```python
from build123d import *

# Parameters (mm, degrees)
SKETCH_1_W           = 88
SKETCH_1_H           = 35
EXTRUDE_1_DEPTH      = 4
EXTRUDE_1_DEPTH_BACK = 4
SKETCH_2_R           = 1.5
CUT_EXTRUDE_1_DEPTH  = 36
EXTRUDE_2_DEPTH      = 12.5


with BuildPart() as part:
    # Sketch 1 → Extrude 1 (new body, two sides)
    with BuildSketch(Plane(origin=(0, 0, 0), x_dir=(1, 0, 0), z_dir=(0, 1, 0))) as extrude_1_sk:
        Rectangle(SKETCH_1_W, SKETCH_1_H)
    extrude(amount=EXTRUDE_1_DEPTH)
    extrude(extrude_1_sk.sketch, amount=-EXTRUDE_1_DEPTH_BACK)

    # Sketch 2 → Cut-Extrude 1 (cut, through all)
    with BuildSketch(Plane(origin=(0, 0, -17.5), x_dir=(-1, 0, 0), z_dir=(0, 0, -1))):
        with Locations((39, 0)):
            Circle(SKETCH_2_R)
        with Locations((-39, 0)):
            Circle(SKETCH_2_R)
        with Locations((-9, 0)):
            Circle(SKETCH_2_R)
        with Locations((9, 0)):
            Circle(SKETCH_2_R)
    extrude(amount=-CUT_EXTRUDE_1_DEPTH, mode=Mode.SUBTRACT)

    # Sketch 3 → Extrude 2 (add, symmetric)
    with BuildSketch(Plane.XY):
        Polygon((29, 4), (22.07179677, 16), (-13.215390309, 16), (-34, 4), align=None)
    extrude(amount=EXTRUDE_2_DEPTH, both=True)


solid = part.part
```
Design review of the part built by this model. Coordinates are the model's own, in mm. A direction names the side the tool comes from. Give positions to 0.01 mm unless a question says otherwise; leave off trailing zeros. Order: outer loops, then holes, each group sorted by start corner. A loop starts at its lowest first (then second) coordinate and runs counter-clockwise, first axis right, second up. Notation, with made-up numbers: M 31.25,44.5 L 62.25,44.5 A27 cw 62.25,68.5 Z; hole C 62,38 d6. An arc over 180 degrees is marked long. One line per question, with ' | ' between items. Start each with the question number.
Q1. For pin 1 Ø9.5 at (x, y) = (7, 8.5) entering from -Z; pin 2 Ø2 at (y, z) = (5.5, 4) entering from +X; pin 3 Ø2 at (y, z) = (9, -11) entering from -X; pin 4 Ø5 at (y, z) = (7, -6.5) entering from -X, all flat-tipped, find the tip position at first contact; note any pin that passes through.
Q2. We need section D-D (x = 9). Write out the cut boundary in (y, z).
Q3. For L1, parallel to Y at x = -9, z = 1; L2, parallel to X at y = -1.25, z = 16.5; L3, parallel to Z at x = -10, y = 5.75, list the stretches that pass through material, from the lowest coordinate up. Write a range as [from, to].
Q4. We need section B-B (z = 4.5). Write out the cut boundary in (x, y).
Q5. The part is to be moulded in two halves that separate along Y. For faces 6 (the face through (-37.8, -0.9, -0.2)), 7 (the face through (10.5, 0.07, -0.25)), 8 (the face through (-1, 0, -17.5)), 9 (the face through (-1, -4, 0)), say which applies: +Y half, -Y half, draft (parallel to the pull), parting line (faces both ways), or undercut.
Q6. We need section A-A (x = -39). Write out the cut boundary in (y, z), plus the area to 3 significant figures.
Q7. We need section C-C (x = -3.5). Write out the cut boundary in (y, z).
Q8. Machinability: for faces 1 (the face through (4, 9, 12.5)), 2 (the face through (25.58, 9.92, 0.18)), 3 (the face through (-1, 4, 15)), 4 (the face through (-1, 0, 17.5)), 5 (the face through (4, 9, -12.5)), which of the approach directions +Z, -Z, +X, -X, +Y, -Y give a long, thin tool a straight path to every point of the face, cutting with its end or side? Answer none if there is none.
Returned:
1) pin 1: z = -17.5 | pin 2: x = 28.71 | pin 3: x = -27.07 | pin 4: x = -33.13
2) outline: M -4,-17.5 L -1.5,-17.5 L -1.5,17.5 L -4,17.5 Z; M 1.5,-17.5 L 4,-17.5 L 4,-12.5 L 16,-12.5 L 16,12.5 L 4,12.5 L 4,17.5 L 1.5,17.5 Z
3) L1: [-4, -1.5], [1.5, 16] | L2: [-44, -39.83], [-38.17, -9.83], [-8.17, 8.17], [9.83, 38.17], [39.83, 44] | L3: [-12.5, 12.5]
4) outline: M -44,-4 L 44,-4 L 44,4 L 29,4 L 22.07,16 L -13.22,16 L -34,4 L -44,4 Z; hole C -39,0 d3; hole C -9,0 d3; hole C 9,0 d3; hole C 39,0 d3
5) face 6: undercut | face 7: undercut | face 8: draft | face 9: -Y half
6) outline: M -4,-17.5 L -1.5,-17.5 L -1.5,17.5 L -4,17.5 Z; M 1.5,-17.5 L 4,-17.5 L 4,17.5 L 1.5,17.5 Z | area: 175 mm2
7) outline: M -4,-17.5 L 4,-17.5 L 4,-12.5 L 16,-12.5 L 16,12.5 L 4,12.5 L 4,17.5 L -4,17.5 Z
8) face 1: +Z, +X, -X, +Y | face 2: +Z, -Z, +X, +Y | face 3: +Y | face 4: +Z, +X, -X, +Y, -Y | face 5: -Z, +X, -X, +Y
